```python
from build123d import *

# Parameters (mm, degrees)
BOSS_EXTRUDE1_DEPTH = 6
SKETCH3_W           = 6.408683363
SKETCH3_H           = 2
SKETCH4_R           = 0.418238454
CUT_EXTRUDE1_DEPTH  = 68.577687393
CUT_EXTRUDE2_DEPTH  = 7.07563293
CUT_EXTRUDE3_DEPTH  = 7.07563293
CUT_EXTRUDE4_DEPTH  = 8.636
SKETCH9_W           = 16.845523319
SKETCH9_H           = 13.536518873
CUT_EXTRUDE5_DEPTH  = 8.636
BOSS_EXTRUDE2_DEPTH = 6
CUT_EXTRUDE6_DEPTH  = 21.59
CUT_EXTRUDE7_DEPTH  = 20.574


with BuildPart() as part:
    # Sketch1 → Boss-Extrude1 (new body)
    with BuildSketch(Plane(origin=(0, 0, 0), x_dir=(1, 0, 0), z_dir=(0, 1, 0))):
        with BuildLine():
            Line((-30.417100683, -25.191255191), (-60.834201366, -25.191255191))
            Line((-60.834201366, -25.191255191), (-60.834201366, -11.654736318))
            Line((-60.834201366, -11.654736318), (-42.452724359, -11.654736318))
            Line((-42.452724359, -11.654736318), (-55.326541771, 11.21298086))
            Line((-55.326541771, 11.21298086), (-24.071247352, 28.808744809))
            Line((-24.071247352, 28.808744809), (-8.250197814, 1.40588318))
            ThreePointArc((-8.250197814, 1.40588318), (-7.349372036, -3.751451104), (-9.988929311, -8.27276965))
            Line((-9.988929311, -8.27276965), (-30.417100683, -25.191255191))
        make_face()
    extrude(amount=BOSS_EXTRUDE1_DEPTH)

    # Sketch3 → Cut-Revolve1 (revolve, cut)
    with BuildSketch(Plane(origin=(0, 0, 0), x_dir=(0.7701644134023178, 0, -0.6378454172671179), z_dir=(0.6378454172671179, 0, 0.7701644134023178))):
        with Locations((-9.738380512, 3)):
            Rectangle(SKETCH3_W, SKETCH3_H)
    revolve(axis=Axis((-5.032284182, 4, 4.167706724), (0, -1, 0)), mode=Mode.SUBTRACT)

    # Sketch4 → Cut-Extrude1 (cut, through all)
    with BuildSketch(Plane(origin=(0, 6, 0), x_dir=(1, 0, 0), z_dir=(0, 1, 0))):
        with Locations(Location((-8.825601509, -4.086499086, 0), (0, 0, 270))):
            Circle(SKETCH4_R)
    extrude(amount=-CUT_EXTRUDE1_DEPTH, mode=Mode.SUBTRACT)

    # Sketch5 → Cut-Extrude2 (cut)
    with BuildSketch(Plane.XZ):
        with BuildLine():
            Line((-24.071247352, -28.808744809), (-10.627789176, 0.89898626))
            ThreePointArc((-10.627789176, 0.89898626), (-8.855926732, 1.209162301), (-7.240059857, 1.999529264))
            ThreePointArc((-7.240059857, 1.999529264), (-7.543928563, 0.237141569), (-8.250197814, -1.40588318))
            Line((-8.250197814, -1.40588318), (-24.071247352, -28.808744809))
        make_face()
    extrude(amount=-CUT_EXTRUDE2_DEPTH, mode=Mode.SUBTRACT)

    # Sketch6 → Cut-Extrude3 (cut)
    with BuildSketch(Plane(origin=(0, 0, 0), x_dir=(-1, 0, 0), z_dir=(0, -1, 0))):
        with BuildLine():
            Line((8.621369431, -1.290415749), (6.275781013, -0.723765639))
            Line((6.275781013, -0.723765639), (7.306606233, -3.4867058))
            ThreePointArc((7.306606233, -3.4867058), (7.684746322, -2.221398672), (8.621369431, -1.290415749))
        make_face()
    extrude(amount=-CUT_EXTRUDE3_DEPTH, mode=Mode.SUBTRACT)

    # Sketch7 → Cut-Extrude4 (cut)
    with BuildSketch(Plane(origin=(0, 6, 0), x_dir=(1, 0, 0), z_dir=(0, 1, 0))):
        Polygon((-9.988929311, -8.27276965), (-29.038929311, -15.05806632), (-29.682744971, -24.58306632), align=None)
    extrude(amount=-CUT_EXTRUDE4_DEPTH, mode=Mode.SUBTRACT)

    # Sketch9 → Cut-Extrude5 (cut)
    with BuildSketch(Plane(origin=(0, 6, 0), x_dir=(1, 0, 0), z_dir=(0, 1, 0))):
        with Locations((-52.411439707, -18.422995755)):
            Rectangle(SKETCH9_W, SKETCH9_H)
    extrude(amount=-CUT_EXTRUDE5_DEPTH, mode=Mode.SUBTRACT)

    # Sketch10 → Boss-Extrude2 (add)
    with BuildSketch(Plane.XZ):
        Polygon((-43.988678047, 11.654736318), (-43.988678047, 8.926427114), (-42.452724359, 11.654736318), align=None)
    extrude(amount=-BOSS_EXTRUDE2_DEPTH)

    # Sketch11 → Cut-Extrude6 (cut)
    with BuildSketch(Plane.XZ):
        Polygon((-55.326541771, -11.21298086), (-43.988678047, 8.926427114), (-26.281813284, -1.041990026), (-37.619677009, -21.181398001), align=None)
    extrude(amount=-CUT_EXTRUDE6_DEPTH, mode=Mode.SUBTRACT)

    # Sketch12 → Cut-Extrude7 (cut)
    with BuildSketch(Plane(origin=(0, 6, 0), x_dir=(1, 0, 0), z_dir=(0, 1, 0))):
        Polygon((-43.988678047, -11.348752844), (-30.168184759, -1.145916898), (-43.988678047, -8.926427114), align=None)
    extrude(amount=-CUT_EXTRUDE7_DEPTH, mode=Mode.SUBTRACT)


solid = part.part
```
Source: CAD feature listing. Evaluate the final solid. Frame: model axes, mm. A direction names the side the tool comes from. Round coordinates to 2 decimals unless told otherwise and drop trailing zeros. Loops run counter-clockwise (first coordinate to the right, second up) from the corner with the lowest first, then second, coordinate; pieces in that order, holes last.
(1) Section query D-D (x = -27.5). Output: boundary loops of the cut face in (y, z).
From the geometry:
outline: (0, -26.88) - (6, -26.88) - (6, -3.21) - (0, -3.21) - close; (0, -0.36) - (6, -0.36) - (6, 14.51) - (0, 14.51) - close
(2) Material intervals for probe 1 along Z at (x, y) = (-28.5, 1.75); probe 2 along Z at (x, y) = (-33, 4.5); probe 3 along Z at (x, y) = (-19, 2.5), sorted ascending.
From the geometry:
probe 1: z = -26.32 to -4.98, 0.21 to 14.87
probe 2: z = -23.78 to -12.98, 3.24 to 25.19
probe 3: z = -17.6 to 11.48
(3) Pull-direction query (Y, two-part tool) for faces 4 (the flat face through (-10, 4, 4)), 5 (the flat face through (-26, 6, -1)), 6 (the flat face through (-19.381, 3.042, 11.618)); classes: +Y half, -Y half, draft (parallel to the pull), parting line (faces both ways), or undercut.
From the geometry:
face 4: undercut
face 5: +Y half
face 6: draft
(4) Contact query for flat-ended pins moving along their axis: pin 1 Ø2 at (x, y) = (-11, 1.5) entering from -Z; pin 2 Ø1.5 at (y, z) = (2.5, 2) entering from +X; pin 3 Ø2 at (x, y) = (-33, 4) entering from -Z; pin 4 Ø4.5 at (x, z) = (-9, 3) entering from -Y. Output: stop coordinate, or through.
From the geometry:
pin 1: stops at z = -2.13
pin 2: stops at x = -7.51
pin 3: stops at z = -24.35
pin 4: stops at y = 0
(5) Section query A-A (x = -35.5). Output: boundary loops of the cut face in (y, z), and give its area (3 significant figures).
From the geometry:
outline: (0, -22.37) - (6, -22.37) - (6, -17.42) - (0, -17.42) - close; (0, 5.08) - (6, 5.08) - (6, 25.19) - (0, 25.19) - close
area: 150 mm2
(6) Access query for faces 1 (the cylindrical face through (-11.417, 3.014, 4.725)), 2 (the flat face through (-28.252, 2.958, 0.067)), 3 (the cylindrical face through (-7.7, 5, 2.2)). Directions: +Z, -Z, +X, -X, +Y, -Y. A direction counts if a zero-diameter tool reaches every point of the face in a straight line with its end or side. Return the directions, or none.
From the geometry:
face 1: +X
face 2: -X, +Y, -Y
face 3: -Z, +X, +Y, -Y
(7) Section query B-B (y = 0.75). Output: boundary loops of the cut face in (x, z).
From the geometry:
outline: (-43.99, 11.35) - (-30.17, 1.15) - (-26.28, -1.04) - (-37.62, -21.18) - (-24.07, -28.81) - (-10.63, 0.9) arc R6.41 ccw to (-8.62, 1.29) arc R2.68 ccw to (-7.31, 3.49) arc R7.62 ccw to (-9.99, 8.27) - (-29.04, 15.06) - (-29.68, 24.58) - (-30.42, 25.19) - (-43.99, 25.19) - close; hole circle Ø0.84 at (-8.83, 4.09)
